Study the drawing (mm; zero at the part's minimum x, y, z) and answer. A direction names the side the tool comes from. Give positions to 0.01 mm unless a question says otherwise; leave off trailing zeros. Loops run counter-clockwise (first coordinate to the right, second up) from the corner with the lowest first, then second, coordinate; pieces in that order, holes last. Notation, with made-up numbers: M 15,74 L 56,74 A25 cw 56,93 Z; hole C -32,-24 d9. An arc over 180 degrees is marked long. Return JSON: item names as keys, results as strings.
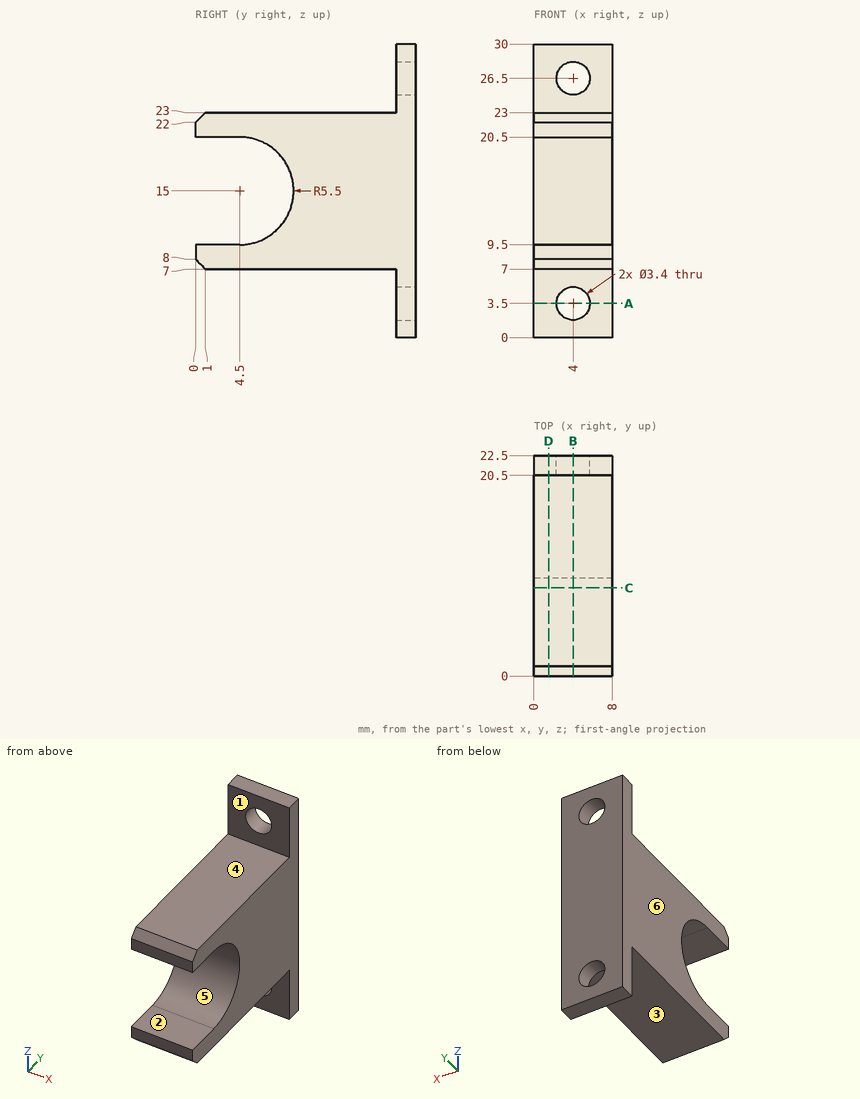
(1) Straight lines are drawn through the part: line 1 along Z through (x, y) = (4, 21.7); line 2 along Z through (x, y) = (3.5, 3.5); line 3 along X through (y, z) = (21.5, 26.5). For each, find the intervals that lie inside material, in ascending order.
Values follow:
{"line 1": "0 to 1.8, 5.2 to 24.8, 28.2 to 30", "line 2": "7 to 9.5, 20.5 to 23", "line 3": "0 to 2.3, 5.7 to 8"}
(2) A tool of negligible diameter and unlimited length cuts with its end or side. For the marked faces 1, 2 and 3, from which of +Z, -Z, +X, -X, +Y, -Y can it reach the whole face along a straight path? Write none if from no direction.
Values follow:
{"face 1": "+Z, +X, -X, -Y", "face 2": "+X, -X, -Y", "face 3": "-Z, +X, -X, -Y"}
(3) Determine the mould class of the marked faces 4, 5 and 6 for opening direction Z: released by +Z, released by -Z, zero draft, split by the parting line, or undercut.
Values follow:
{"face 4": "released by +Z", "face 5": "undercut", "face 6": "zero draft"}
(4) The part is cut by section A-A (z = 3.5). Determine the outline of the cut face in (x, y), and give its area (3 significant figures).
Values follow:
{"outline": "M 0,20.5 L 2.3,20.5 L 2.3,22.5 L 0,22.5 Z; M 5.7,20.5 L 8,20.5 L 8,22.5 L 5.7,22.5 Z", "area": "9.20 mm²"}
(5) The part is cut by section B-B (x = 4). Determine the outline of the cut face in (y, z).
Values follow:
{"outline": "M 0,8 L 1,7 L 20.5,7 L 20.5,5.2 L 22.5,5.2 L 22.5,24.8 L 20.5,24.8 L 20.5,23 L 1,23 L 0,22 L 0,20.5 L 4.5,20.5 A5.5 cw 4.5,9.5 L 0,9.5 Z; M 20.5,0 L 22.5,0 L 22.5,1.8 L 20.5,1.8 Z; M 20.5,28.2 L 22.5,28.2 L 22.5,30 L 20.5,30 Z"}
(6) The part is cut by section C-C (y = 9). Determine the outline of the cut face in (x, z).
Values follow:
{"outline": "M 0,7 L 8,7 L 8,11.84 L 0,11.84 Z; M 0,18.16 L 8,18.16 L 8,23 L 0,23 Z"}
(7) The part is cut by section D-D (x = 1.5). Determine the outline of the cut face in (y, z), and give its area (3 significant figures).
Values follow:
{"outline": "M 0,8 L 1,7 L 20.5,7 L 20.5,0 L 22.5,0 L 22.5,30 L 20.5,30 L 20.5,23 L 1,23 L 0,22 L 0,20.5 L 4.5,20.5 A5.5 cw 4.5,9.5 L 0,9.5 Z", "area": "290 mm²"}
(8) Given pin 1 (1.3 mm diameter, centred on x = 4.5, y = 1.5, fed in from +Z); pin 2 (6 mm diameter, centred on y = 11.5, z = 12.5, fed in from -X); pin 3 (3 mm diameter, centred on x = 4, z = 3.5, fed in from -Y); pin 4 (4 mm diameter, centred on x = 5, z = 18, fed in from -Y), each flat-ended and moving along its own axis, determine where each tip first touches the part or whether it passes through.
Values follow:
{"pin 1": "z = 23", "pin 2": "x = 0", "pin 3": "through", "pin 4": "y = 6.79"}
